Part model, mm, in its own coordinate system. Give positions to 0.01 mm unless a question says otherwise; leave off trailing zeros. Loops run counter-clockwise (first coordinate to the right, second up) from the corner with the lowest first, then second, coordinate; pieces in that order, holes last. Notation, with made-up numbers: (-39, 15) -> (7, 15) arc R14 ccw to (7, 27) -> close; hole circle Ø4 at (71.5, 68.25). An arc over 180 degrees is marked (long way). One line per question, with ' | ' between items.
```python
from build123d import *

# Parameters (mm, degrees)
SKETCH1_W                = 75
SKETCH1_H                = 160
BOSS_EXTRUDE1_DEPTH      = 3
M3_CLEARANCE_HOLE1_D     = 3.4
M3_CLEARANCE_HOLE1_DEPTH = 3
M3_CLEARANCE_HOLE1_TIP   = 1.021463052
SKETCH6_W                = 3
SKETCH6_H                = 10
SKETCH6_H_2              = 15.175339059
CUT_EXTRUDE3_DEPTH       = 10
SKETCH7_W                = 3
SKETCH7_H                = 10
CUT_EXTRUDE4_DEPTH       = 10


with BuildPart() as part:
    # Sketch1 → Boss-Extrude1 (new body)
    with BuildSketch(Plane(origin=(0, 0, 0), x_dir=(1, 0, 0), z_dir=(0, 1, 0))):
        with Locations((37.5, 80)):
            Rectangle(SKETCH1_W, SKETCH1_H)
    extrude(amount=BOSS_EXTRUDE1_DEPTH)

    # M3 Clearance Hole1
    with Locations(Plane(origin=(0, 0, 0), x_dir=(-1, 0, 0), z_dir=(0, -1, 0))):
        with Locations((-68.5, 19), (-56, 55.55), (-56, 34.55), (-6.5, 19), (-61, 139.5), (-14, 139.5), (-6.5, 100), (-68.5, 100)):
            Hole(M3_CLEARANCE_HOLE1_D / 2, depth=M3_CLEARANCE_HOLE1_DEPTH)
            with Locations((0, 0, -(M3_CLEARANCE_HOLE1_DEPTH + M3_CLEARANCE_HOLE1_TIP / 2))):  # 118° drill point
                Cone(0, M3_CLEARANCE_HOLE1_D / 2, M3_CLEARANCE_HOLE1_TIP, mode=Mode.SUBTRACT)

    # Sketch6 → Cut-Extrude3 (cut)
    with BuildSketch(Plane.XZ):
        with Locations((61, -149.447708573)):
            Rectangle(SKETCH6_W, SKETCH6_H)
        with Locations((61, -126.680039044)):
            Rectangle(SKETCH6_W, SKETCH6_H_2)
        with Locations((14, -149.447708573)):
            Rectangle(SKETCH6_W, SKETCH6_H)
        with Locations((14, -126.680039044)):
            Rectangle(SKETCH6_W, SKETCH6_H_2)
    extrude(amount=-CUT_EXTRUDE3_DEPTH, mode=Mode.SUBTRACT)

    # Sketch7 → Cut-Extrude4 (cut)
    with BuildSketch(Plane.XZ):
        with Locations((6.5, -9)):
            Rectangle(SKETCH7_W, SKETCH7_H)
        with Locations((6.5, -29)):
            Rectangle(SKETCH7_W, SKETCH7_H)
        with Locations((68.5, -29)):
            Rectangle(SKETCH7_W, SKETCH7_H)
        with Locations((68.5, -9)):
            Rectangle(SKETCH7_W, SKETCH7_H)
        with Locations((56, -45)):
            Rectangle(SKETCH7_W, SKETCH7_H)
        with Locations((6.5, -90)):
            Rectangle(SKETCH7_W, SKETCH7_H)
        with Locations((68.5, -90)):
            Rectangle(SKETCH7_W, SKETCH7_H)
    extrude(amount=-CUT_EXTRUDE4_DEPTH, mode=Mode.SUBTRACT)


solid = part.part
```
1) Saw through at D-D (x = 6.5). Give the cut face in (y, z).
Found:
outline: (0, -160) -> (3, -160) -> (3, -101.7) -> (0, -101.7) -> close; (0, -98.3) -> (3, -98.3) -> (3, -95) -> (0, -95) -> close; (0, -85) -> (3, -85) -> (3, -34) -> (0, -34) -> close; (0, -24) -> (3, -24) -> (3, -20.7) -> (0, -20.7) -> close; (0, -17.3) -> (3, -17.3) -> (3, -14) -> (0, -14) -> close; (0, -4) -> (3, -4) -> (3, 0) -> (0, 0) -> close
2) Saw through at B-B (x = 56). Give the cut face in (y, z), and give its area (3 significant figures).
Found:
outline: (0, -160) -> (3, -160) -> (3, -57.25) -> (0, -57.25) -> close; (0, -53.85) -> (3, -53.85) -> (3, -50) -> (0, -50) -> close; (0, -40) -> (3, -40) -> (3, -36.25) -> (0, -36.25) -> close; (0, -32.85) -> (3, -32.85) -> (3, 0) -> (0, 0) -> close | area: 430 mm2
3) Pull direction Z, two halves, no side cores. Call faces 1 (the flat face through (8, 1, -29)), 2 (the flat face through (0, 1, -79)), 3 (the flat face through (37, 1, 0)), 4 (the cylindrical face through (59.3, 1.52, -139.57)): pulls with the +Z half, pulls with the -Z half, needs draft (parallel to the pull), parting line crosses it, or undercut.
Found:
face 1: undercut | face 2: needs draft | face 3: pulls with the +Z half | face 4: undercut
4) Drill centre lines: line 1 (Z direction, x = 68.5, y = 1.4); line 2 (X direction, y = 0.75, z = -89.5); line 3 (X direction, y = 0.6, z = -100). Where is each one in solid material? Low to high.
Found:
line 1: -160 to -101.7, -98.3 to -95, -85 to -34, -24 to -20.7, -17.3 to -14, -4 to 0 | line 2: 0 to 5, 8 to 67, 70 to 75 | line 3: 0 to 4.8, 8.2 to 66.8, 70.2 to 75
5) Saw through at A-A (z = -100). Give the cut face in (x, y), and give its area (3 significant figures).
Found:
outline: (0, 0) -> (4.8, 0) -> (4.8, 3) -> (0, 3) -> close; (8.2, 0) -> (66.8, 0) -> (66.8, 3) -> (8.2, 3) -> close; (70.2, 0) -> (75, 0) -> (75, 3) -> (70.2, 3) -> close | area: 205 mm2
6) Saw through at C-C (z = -55.55). Give the cut face in (x, y), and give its area (3 significant figures).
Found:
outline: (0, 0) -> (54.3, 0) -> (54.3, 3) -> (0, 3) -> close; (57.7, 0) -> (75, 0) -> (75, 3) -> (57.7, 3) -> close | area: 215 mm2
